from build123d import *

# Parameters (mm, degrees)
F1_DEPTH = 12.5
F2_R     = 20


with BuildPart() as f1:
    # F0 (on Front) → F1 (new body, symmetric)
    with BuildSketch(Plane.XZ):
        with BuildLine():
            add(Edge.make_bspline(
                [(0, 230), (-143.18813182, 115), (0, 0)],
                knots=[5.8897826752, 5.8897826752, 5.8897826752, 6.6765879392, 6.6765879392, 6.6765879392], degree=2, weights=[1, 0.9236100668, 1]))
            Line((0, 0), (1150, 0))
            Line((1150, 0), (1150, 25))
            Line((1150, 25), (9.1600259417, 25))
            add(Edge.make_bspline(
                [(9.1600259417, 205), (-89.4541344002, 115), (9.1600259417, 25)],
                knots=[5.949769397, 5.949769397, 5.949769397, 6.6166012174, 6.6166012174, 6.6166012174], degree=2, weights=[1, 0.9449299244, 1]))
            Line((9.1600259417, 205), (350, 205))
            Line((350, 205), (350, 230))
            Line((350, 230), (0, 230))
        make_face()
    extrude(amount=F1_DEPTH, both=True)

    # F2
    f2_edges = [f1.edges().sort_by_distance(p)[0] for p in [
        (9.160026, -6.25, 25),
        (9.160026, 6.25, 25),
        (9.160026, -6.25, 205),
        (9.160026, 6.25, 205),
    ]]
    fillet(f2_edges, radius=F2_R)


solid = f1.part
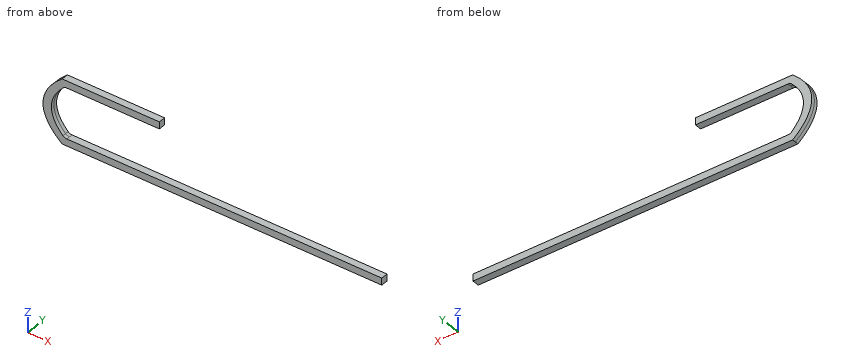
Part model, mm, in its own coordinate system. Coordinates: 2 decimals unless noted, no trailing zeros. Order: outer loops, then holes, each group sorted by start corner. A loop starts at its lowest first (then second) coordinate and runs counter-clockwise, first axis right, second up. Notation, with made-up numbers: (51, 8) - (56, 8) arc R13 cw to (56, 13) - close; hole circle Ø6 at (48.25, 18.25). An arc over 180 degrees is marked (long way). Use CSV: the item, a comma, the result in double quotes.
Item 1: Drop flat-ended pins along their axis: P1, Ø12, axis at x = 334, y = 8.5, coming from the -Z side; P2, Ø12.5, axis at x = 656, y = -1, coming from the +Z side; P3, Ø5, axis at y = -2, z = 158, coming from the -X side; P4, Ø8, axis at y = -4.5, z = 149.5, coming from the -X side. Give the stop position or say it passes through.
Solved:
P1,"stops at z = 0"
P2,"stops at z = 25"
P3,"stops at x = -60.51"
P4,"stops at x = -64.09"
Item 2: Probe probe 1 along Z at (x, y) = (49, -0.75); probe 2 along Z at (x, y) = (822, 4.75); probe 3 along X at (y, z) = (10, 117.5). List the from-to ranges inside material, lowest first.
Solved:
probe 1,"z = 0 to 25, 205 to 230"
probe 2,"z = 0 to 25"
probe 3,"x = -68.72 to -38.71"
Item 3: Saw through at B-B on x = 634.5. Give the cut face in (y, z).
Solved:
outline,"(-12.5, 0) - (12.5, 0) - (12.5, 25) - (-12.5, 25) - close"
Item 4: Saw through at A-A on x = 242.5. Give the cut face in (y, z), and give its area (3 significant figures).
Solved:
outline,"(-12.5, 0) - (12.5, 0) - (12.5, 25) - (-12.5, 25) - close; (-12.5, 205) - (12.5, 205) - (12.5, 230) - (-12.5, 230) - close"
area,"1,250 mm²"
